from build123d import *

# Parameters (mm, degrees)
SKETCH1_W               = 406.4
SKETCH1_H               = 508
BOSS_EXTRUDE1_DEPTH     = 3.175
SKETCH2_R               = 14.2875
CUT_EXTRUDE1_DEPTH      = 3.175
SKETCH3_R               = 2.4892
CUT_EXTRUDE2_DEPTH      = 1
CUT_EXTRUDE2_DEPTH_BACK = 4.175
SKETCH4_R               = 2.413
CUT_EXTRUDE3_DEPTH      = 1
CUT_EXTRUDE3_DEPTH_BACK = 4.175


with BuildPart() as part:
    # Sketch1 → Boss-Extrude1 (new body)
    with BuildSketch(Plane(origin=(0, 0, 0), x_dir=(1, 0, 0), z_dir=(0, 1, 0))):
        with Locations((203.2, 254)):
            Rectangle(SKETCH1_W, SKETCH1_H)
    extrude(amount=BOSS_EXTRUDE1_DEPTH)

    # Sketch2 → Cut-Extrude1 (cut)
    with BuildSketch(Plane(origin=(0, 3.175, 0), x_dir=(1, 0, 0), z_dir=(0, 1, 0))):
        with Locations((50.8, 419.1)):
            Circle(SKETCH2_R)
        with Locations((165.1, 419.1)):
            Circle(SKETCH2_R)
        with Locations((50.8, 88.9)):
            Circle(SKETCH2_R)
        with Locations((165.1, 88.9)):
            Circle(SKETCH2_R)
    extrude(amount=-CUT_EXTRUDE1_DEPTH, mode=Mode.SUBTRACT)

    # Sketch3 → Cut-Extrude2 (cut, two sides)
    with BuildSketch(Plane(origin=(0, 3.175, 0), x_dir=(1, 0, 0), z_dir=(0, 1, 0))) as cut_extrude2_sk:
        with Locations((38.1, 12.7)):
            Circle(SKETCH3_R)
        with Locations((63.5, 12.7)):
            Circle(SKETCH3_R)
        with Locations((127, 12.7)):
            Circle(SKETCH3_R)
        with Locations((152.4, 12.7)):
            Circle(SKETCH3_R)
        with Locations((177.8, 12.7)):
            Circle(SKETCH3_R)
        with Locations((203.2, 12.7)):
            Circle(SKETCH3_R)
        with Locations((228.6, 12.7)):
            Circle(SKETCH3_R)
        with Locations((254, 12.7)):
            Circle(SKETCH3_R)
        with Locations((279.4, 12.7)):
            Circle(SKETCH3_R)
        with Locations((304.8, 12.7)):
            Circle(SKETCH3_R)
        with Locations((330.2, 12.7)):
            Circle(SKETCH3_R)
        with Locations((355.6, 12.7)):
            Circle(SKETCH3_R)
        with Locations((381, 12.7)):
            Circle(SKETCH3_R)
        with Locations((381, 495.3)):
            Circle(SKETCH3_R)
        with Locations((355.6, 495.3)):
            Circle(SKETCH3_R)
        with Locations((330.2, 495.3)):
            Circle(SKETCH3_R)
        with Locations((304.8, 495.3)):
            Circle(SKETCH3_R)
        with Locations((279.4, 495.3)):
            Circle(SKETCH3_R)
        with Locations((254, 495.3)):
            Circle(SKETCH3_R)
        with Locations((228.6, 495.3)):
            Circle(SKETCH3_R)
        with Locations((203.2, 495.3)):
            Circle(SKETCH3_R)
        with Locations((177.8, 495.3)):
            Circle(SKETCH3_R)
        with Locations((152.4, 495.3)):
            Circle(SKETCH3_R)
        with Locations((127, 495.3)):
            Circle(SKETCH3_R)
        with Locations((63.5, 495.3)):
            Circle(SKETCH3_R)
        with Locations((38.1, 495.3)):
            Circle(SKETCH3_R)
        with Locations((101.6, 12.7)):
            Circle(SKETCH3_R)
    extrude(amount=CUT_EXTRUDE2_DEPTH, mode=Mode.SUBTRACT)
    extrude(cut_extrude2_sk.sketch, amount=-CUT_EXTRUDE2_DEPTH_BACK, mode=Mode.SUBTRACT)

    # Sketch4 → Cut-Extrude3 (cut, two sides)
    with BuildSketch(Plane.XZ) as cut_extrude3_sk:
        with Locations((38.179625472, -334.938702735)):
            Circle(SKETCH4_R)
        with Locations((63.579625472, -334.938702735)):
            Circle(SKETCH4_R)
        with Locations((63.579625472, -360.338702735)):
            Circle(SKETCH4_R)
        with Locations((38.179625472, -360.338702735)):
            Circle(SKETCH4_R)
        with Locations((63.461499211, -173.060090351)):
            Circle(SKETCH4_R)
        with Locations((38.061499211, -173.060090351)):
            Circle(SKETCH4_R)
        with Locations((38.061499211, -147.660090351)):
            Circle(SKETCH4_R)
        with Locations((63.461499211, -147.660090351)):
            Circle(SKETCH4_R)
    extrude(amount=CUT_EXTRUDE3_DEPTH, mode=Mode.SUBTRACT)
    extrude(cut_extrude3_sk.sketch, amount=-CUT_EXTRUDE3_DEPTH_BACK, mode=Mode.SUBTRACT)


solid = part.part
CAD build for the part. Positions are in the model's coordinates, mm. Round coordinates to 2 decimals unless told otherwise and drop trailing zeros. Use one line per item in the form item = value.
Q1. Flat gauge pin, fed straight in: P1, Ø4, axis at x = 279.4, z = -12.7, coming from the +Y side. Where does the tip first touch, or does it go through?
Recorded:
P1 = through
Q2. Two-plate mould, pull along X, no slides. Class faces 1 (the cylindrical face through (172.78, 1.61, -431.15)), 2 (the flat face through (200, 0, -258)): +X half, -X half, draft (parallel to the pull), parting line (faces both ways), or undercut.
Recorded:
face_1 = undercut
face_2 = draft
Q3. Saw through at A-A on y = 1.7. State how many separate pieces and enclosed holes the cut face has, then the cut area to 3 significant figures.
Recorded:
separate_pieces = 1
enclosed_holes = 39
area = 203,000 mm^2
Q4. Probe L1, parallel to Z at x = 50.8, y = 1.55; L2, parallel to Z at x = 355, y = 1.05; L3, parallel to Z at x = 101.6, y = 2.1. List the from-to ranges inside material, lowest first.
Recorded:
L1 = -508 to -433.39, -404.81 to -103.19, -74.61 to 0
L2 = -508 to -497.72, -492.88 to -15.12, -10.28 to 0
L3 = -508 to -15.19, -10.21 to 0
